Design review of the part built by this model. Coordinates are the model's own, in mm. Face numbers are marked on the shaded views. A direction names the side the tool comes from. Give positions to 0.01 mm unless a question says otherwise; leave off trailing zeros. Write each loop counter-clockwise with the first axis right and the second up, starting at its lowest first coordinate (ties: lowest second). Pieces come first, ordered by that corner, then holes. Notation, with made-up numbers: M 19.5,0 L 61.5,0 A25 cw 61.5,39 Z; hole C 6,-27.75 d11. An arc over 180 degrees is marked long. Write each question's results on one line, items separated by ' | '. Start each with the question number.
from build123d import *

# Parameters (mm, degrees)
F0_R     = 0.8
F0_R_2   = 5
F1_DEPTH = 45.5
F2_W     = 39.5
F2_H     = 30
F3_DEPTH = 20.001
F4_DEPTH = 45.501
F5_R     = 5


with BuildPart() as f1:
    # F0 (on Front) → F1 (new body)
    with BuildSketch(Plane.XZ):
        with BuildLine():
            ThreePointArc((-2.67e-08, 10), (-7.0710678213, 7.0710678024), (-10, 0))
            ThreePointArc((-10, 0), (0, -10), (10, 0))
            ThreePointArc((10, 0), (7.0710678024, 7.0710678213), (-2.67e-08, 10))
        make_face()
        with Locations((-7, 0)):
            Circle(F0_R, mode=Mode.SUBTRACT)
        with Locations((-4.9497474683, -4.9497474683)):
            Circle(F0_R, mode=Mode.SUBTRACT)
        with Locations((0, -7)):
            Circle(F0_R, mode=Mode.SUBTRACT)
        with Locations((4.9497474683, -4.9497474683)):
            Circle(F0_R, mode=Mode.SUBTRACT)
        Circle(F0_R_2, mode=Mode.SUBTRACT)
        with Locations((7, 0)):
            Circle(F0_R, mode=Mode.SUBTRACT)
        with Locations((0, 7)):
            Circle(F0_R, mode=Mode.SUBTRACT)
        with BuildLine():
            ThreePointArc((10, 0), (0, -10), (-10, 0))
            Line((-10, 0), (-10, -22))
            Line((-10, -22), (10, -22))
            Line((10, -22), (10, 0))
        make_face()
        Circle(F0_R_2)
        Polygon((10, -22), (-10, -22), (-10, -25), (0, -25), (10, -25), align=None)
        with BuildLine():
            ThreePointArc((-2.67e-08, 10), (7.0710678024, 7.0710678213), (10, 0))
            Line((10, 0), (10, 10))
            Line((10, 10), (-2.67e-08, 10))
        make_face()
        with BuildLine():
            Line((-10, 10), (-10, 0))
            ThreePointArc((-10, 0), (-7.0710678213, 7.0710678024), (-2.67e-08, 10))
            Line((-2.67e-08, 10), (-10, 10))
        make_face()
        with Locations((0, -7)):
            Circle(F0_R)
        with Locations((7, 0)):
            Circle(F0_R)
        with Locations((-4.9497474683, -4.9497474683)):
            Circle(F0_R)
        with Locations((-7, 0)):
            Circle(F0_R)
        with Locations((0, 7)):
            Circle(F0_R)
        with Locations((4.9497474683, -4.9497474683)):
            Circle(F0_R)
    extrude(amount=-F1_DEPTH)

    # F2 (on face) → F3 (cut, through all)
    with BuildSketch(Plane.YZ.offset(10)):
        with Locations((22.75, -5)):
            Rectangle(F2_W, F2_H)
    extrude(amount=-F3_DEPTH, mode=Mode.SUBTRACT)

    # F0 (on Front) → F4 (cut, through all)
    with BuildSketch(Plane.XZ):
        Circle(F0_R_2)
        with BuildLine():
            Line((-10, 10), (-10, 0))
            ThreePointArc((-10, 0), (-7.0710678213, 7.0710678024), (-2.67e-08, 10))
            Line((-2.67e-08, 10), (-10, 10))
        make_face()
        with BuildLine():
            ThreePointArc((-2.67e-08, 10), (7.0710678024, 7.0710678213), (10, 0))
            Line((10, 0), (10, 10))
            Line((10, 10), (-2.67e-08, 10))
        make_face()
        with Locations((7, 0)):
            Circle(F0_R)
        with Locations((0, 7)):
            Circle(F0_R)
        with Locations((-7, 0)):
            Circle(F0_R)
        with Locations((-4.9497474683, -4.9497474683)):
            Circle(F0_R)
        with Locations((0, -7)):
            Circle(F0_R)
        with Locations((4.9497474683, -4.9497474683)):
            Circle(F0_R)
    extrude(amount=-F4_DEPTH, mode=Mode.SUBTRACT)

    # F5
    f5_edges = [f1.edges().sort_by_distance(p)[0] for p in [
        (0, 42.5, -20),
        (0, 3, -20),
    ]]
    fillet(f5_edges, radius=F5_R)


solid = f1.part
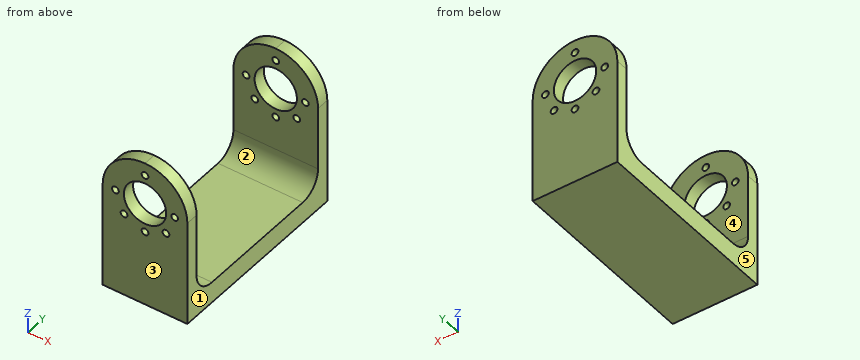
Q1. Wall thickness on line 1 along Y through (x, z) = (4, 5.5); line 2 along Z through (x, y) = (-4, 24); line 3 along Y through (x, z) = (-2, -17): over which ranges is each line inside the solid? List them lowest first. Write a range as from..to.
Q2. We need section B-B on z = -15.5. Write out the cut boundary in (x, y).
Q3. We need section D-D on y = 26. Write out the cut boundary in (x, z).
Q4. For the marked faces 1 and 2, list the 3-axis set-ups (+Z, -Z, +X, -X, +Y, -Y) from which the entire face can be reached by the end or side of a thin tool; tool diameter is ignored.
Q5. The part is to be moulded in two halves that separate along Y. For the marked faces 3, 4 and 5, say which applies: pulls with the +Y half, pulls with the -Y half, needs draft (parallel to the pull), parting line crosses it, or undercut.
Q6. For pin 1 Ø12 at (x, y) = (7, 20) entering from +Z; pin 2 Ø2.5 at (x, z) = (-4.95, -4.95) entering from +Y; pin 3 Ø10 at (x, y) = (5, 6) entering from +Z; pin 4 Ø10 at (x, y) = (8, 35) entering from +Z, all flat-tipped, find the tip position at first contact; note any pin that passes through.
Q7. We need section A-A on z = -3. Write out the cut boundary in (x, y).
Q8. We need section C-C on x = 2. Write out the cut boundary in (y, z).
Answer sheet:
1) line 1: 0..3, 42.5..45.5 | line 2: -25..-20 | line 3: 0..3.42, 42.08..45.5
2) outline: M -10,0 L 10,0 L 10,3.03 L -10,3.03 Z; M -10,42.47 L 10,42.47 L 10,45.5 L -10,45.5 Z
3) outline: M -10,-25 L 10,-25 L 10,-20 L -10,-20 Z
4) face 1: +Z, -Z, +X, +Y, -Y | face 2: +Z, +X, -X
5) face 3: pulls with the -Y half | face 4: undercut | face 5: needs draft
6) pin 1: z = -20 | pin 2: y = 45.5 | pin 3: z = 9.95 | pin 4: z = -19.33
7) outline: M -10,0 L -4,0 L -4,3 L -10,3 Z; M -10,42.5 L -4,42.5 L -4,45.5 L -10,45.5 Z; M 4,0 L 10,0 L 10,3 L 4,3 Z; M 4,42.5 L 10,42.5 L 10,45.5 L 4,45.5 Z
8) outline: M 0,-25 L 45.5,-25 L 45.5,-4.58 L 42.5,-4.58 L 42.5,-15 A5 cw 37.5,-20 L 8,-20 A5 cw 3,-15 L 3,-4.58 L 0,-4.58 Z; M 0,4.58 L 3,4.58 L 3,9.8 L 0,9.8 Z; M 42.5,4.58 L 45.5,4.58 L 45.5,9.8 L 42.5,9.8 Z
